The drawing under review shows one solid part. Ordinate dimensions are in mm from its lowest x, y, z. A direction names the side the tool comes from. Give positions to 0.01 mm unless a question says otherwise; leave off trailing zeros. Order: outer loops, then holes, each group sorted by start corner. A loop starts at its lowest first (then second) coordinate and runs counter-clockwise, first axis right, second up. Notation, with made-up numbers: (52.5, -32.75) - (101.5, -32.75) arc R20 cw to (101.5, -13.75) - close; hole circle Ø5 at (-30.75, 20). An arc over 180 degrees is marked (long way). Answer as a JSON object with one key per item and string values. Group by question number.
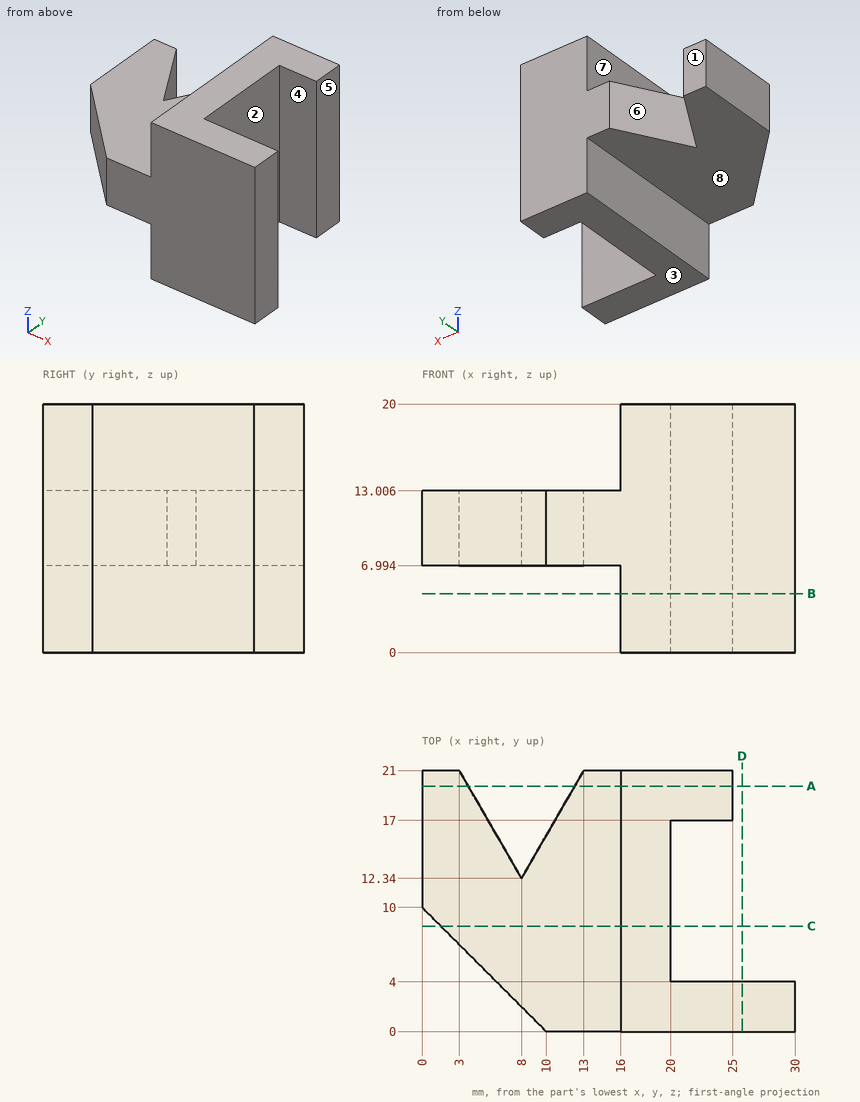
1) Consider section D-D (x = 25.75). Give the boundary of the cut face in (y, z), plus the area to 3 significant figures.
2) Mouldability with a two-part tool opening along Y and no side actions: class the marked faces 1, 2 and 3 as released by +Y, released by -Y, zero draft, split by the parting line, or undercut.
3) Consider section A-A (y = 19.75). Give the boundary of the cut face in (x, z) (1 decimal), plus the area to 3 significant figures.
4) For pin 1 (2 mm diameter, centred on x = 25.5, y = 19, fed in from +Z); pin 2 (1 mm diameter, centred on x = 12, y = 6, fed in from -Z); pin 3 (7.5 mm diameter, centred on y = 9.5, z = 3, fed in from -X); pin 4 (3 mm diameter, centred on y = 6.5, z = 6, fed in from +X), all flat-tipped, find the tip position at first contact; note any pin that passes through.
5) Consider section C-C (y = 8.5). Give the boundary of the cut face in (x, z) (1 decimal).
6) For line 1 (X direction, y = 10.5, z = 19); line 2 (X direction, y = 3, z = 16); line 3 (Z direction, x = 14, y = 4.75) (1 decimal), list the stretches that pass through material, from the lowest coordinate up.
7) Consider section B-B (z = 4.75). Give the boundary of the cut face in (x, y).
8) For the marked faces 4, 5, 6, 7 and 8, list the 3-axis set-ups (+Z, -Z, +X, -X, +Y, -Y) from which the entire face can be reached by the end or side of a thin tool; tool diameter is ignored.
Result set:
{
 "1": {"outline": "(0, 0) - (4, 0) - (4, 20) - (0, 20) - close", "area": "80.0 mm2"},
 "2": {"face 1": "released by +Y", "face 2": "undercut", "face 3": "zero draft"},
 "3": {"outline": "(0, 7) - (3.7, 7) - (3.7, 13) - (0, 13) - close; (12.3, 7) - (16, 7) - (16, 0) - (25, 0) - (25, 20) - (16, 20) - (16, 13) - (12.3, 13) - close", "area": "225 mm2"},
 "4": {"pin 1": "stops at z = 20", "pin 2": "stops at z = 6.99", "pin 3": "stops at x = 16", "pin 4": "stops at x = 20"},
 "5": {"outline": "(1.5, 7) - (16, 7) - (16, 0) - (20, 0) - (20, 20) - (16, 20) - (16, 13) - (1.5, 13) - close"},
 "6": {"line 1": "x = 16 to 20", "line 2": "x = 16 to 30", "line 3": "z = 7 to 13"},
 "7": {"outline": "(16, 0) - (30, 0) - (30, 4) - (20, 4) - (20, 17) - (25, 17) - (25, 21) - (16, 21) - close"},
 "8": {"face 4": "+Z, -Z, +X", "face 5": "+Z, -Z, +X, +Y", "face 6": "+Z, -Z, +Y", "face 7": "+Z, -X, +Y, -Y", "face 8": "-Z, -X, +Y, -Y"}
}
